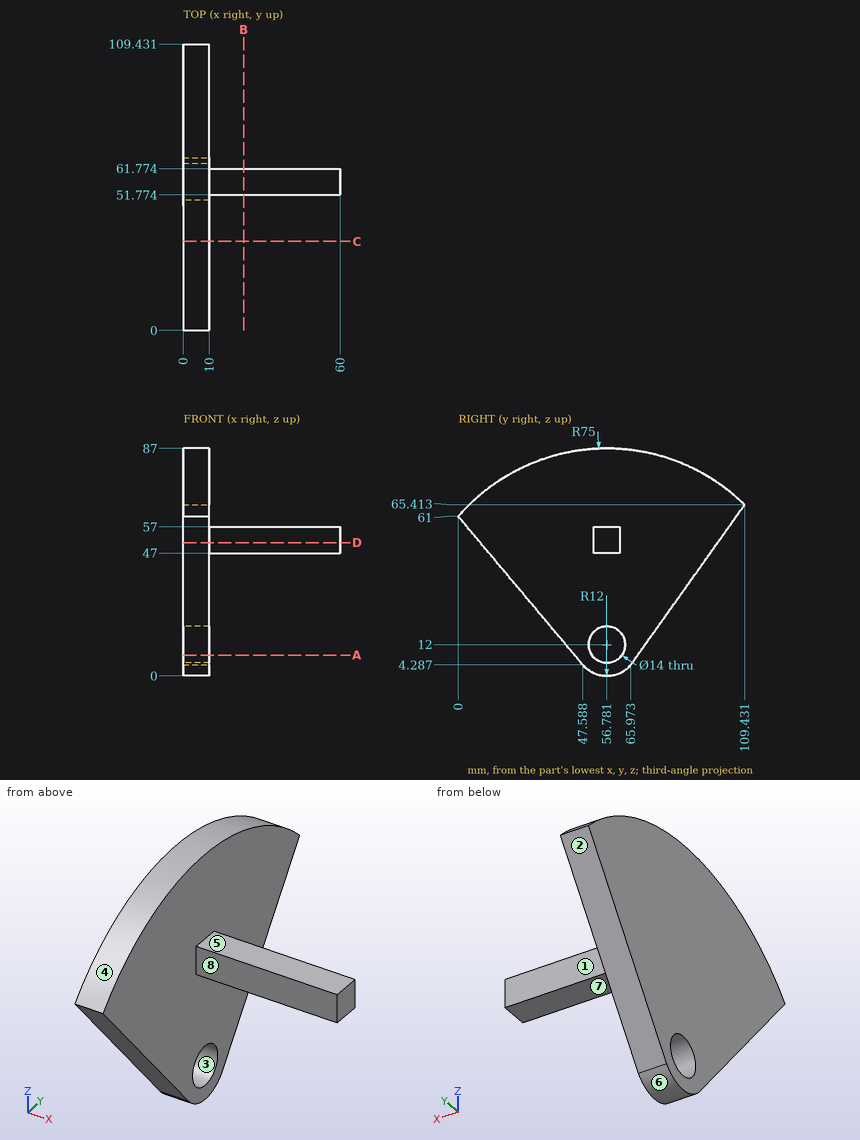
For this review, use the dimensioned drawing (mm, ordinates from the lowest corner) and the shaded views. A direction names the side the tool comes from. Coordinates: 2 decimals unless noted, no trailing zeros. Loops run counter-clockwise (first coordinate to the right, second up) from the corner with the lowest first, then second, coordinate; pieces in that order, holes last. Notation, with made-up numbers: (8.25, 63.5) - (15.25, 63.5) arc R17 cw to (15.25, 95.5) - close; hole circle Ø11 at (36, 62.25). An arc over 180 degrees is marked (long way). Use CSV: the item, a comma, the result in double quotes. Start each with the question number.
1) Consider section C-C on y = 34. Write out the cut boundary in (x, z), then the cut area to 3 significant figures.
2) Tool access review of the marked faces 5, 6, 7 and 8: name each direction out of +Z, -Z, +X, -X, +Y, -Y from which nothing blocks a thin tool from reaching the whole face with its end or side.
3) Consider section B-B on x = 23. Write out the cut boundary in (y, z) (1 decimal).
4) The part is to be moulded in two halves that separate along Z. For the marked faces 1, 2, 3 and 4, say which applies: +Z half, -Z half, draft (parallel to the pull), parting line (faces both ways), or undercut.
5) For pin 1 Ø12 at (y, z) = (41, 44.5) entering from +X; pin 2 Ø10 at (x, y) = (12, 88.5) entering from -Z (1 decimal); pin 3 Ø3 at (x, y) = (31, 57.5) entering from -Z, all flat-tipped, find the tip position at first contact; note any pin that passes through.
6) Consider section A-A on z = 8. Write out the cut boundary in (x, y) (1 decimal).
7) Wall thickness on L1, parallel to X at y = 45, z = 63; L2, parallel to Y at x = 5, z = 11.5 (1 decimal); L3, parallel to Z at x = 28.5, y = 58.5: over which ranges is each line inside the solid? List them lowest first. Write a range as from..to.
8) Consider section D-D on z = 51. Write out the cut boundary in (x, y) (1 decimal).
Geometry says:
1,outline,"(0, 20.48) - (10, 20.48) - (10, 83.46) - (0, 83.46) - close"
1,area,"630 mm^2"
2,face 5,"+Z, +X, +Y, -Y"
2,face 6,"-Z, +X, -X"
2,face 7,"-Z, +X, +Y, -Y"
2,face 8,"+Z, -Z, +X, -Y"
3,outline,"(51.8, 47) - (61.8, 47) - (61.8, 57) - (51.8, 57) - close"
4,face 1,"draft"
4,face 2,"-Z half"
4,face 3,"undercut"
4,face 4,"+Z half"
5,pin 1,"x = 10"
5,pin 2,"z = 29.5"
5,pin 3,"z = 47"
6,outline,"(0, 44.5) - (10, 44.5) - (10, 51) - (0, 51) - close; (0, 62.5) - (10, 62.5) - (10, 68.6) - (0, 68.6) - close"
7,L1,"0..10"
7,L2,"41.5..49.8, 63.8..71.1"
7,L3,"47..57"
8,outline,"(0, 8.4) - (10, 8.4) - (10, 51.8) - (60, 51.8) - (60, 61.8) - (10, 61.8) - (10, 99.2) - (0, 99.2) - close"
